```python
from build123d import *

# Parameters (mm, degrees)
F3_R     = 1.55
F4_DEPTH = 21.928203
F7_DEPTH = 4


with BuildPart() as f2:
    # F1 (on Front) → F2 (revolve)
    with BuildSketch(Plane.XZ):
        with BuildLine():
            Line((-4, -6.928203), (-4, -13.928203))
            Line((-4, -13.928203), (0, -13.928203))
            Line((0, -13.928203), (0, 8))
            ThreePointArc((0, 8), (-7.727407, 2.070552), (-4, -6.928203))
        make_face()
    revolve(axis=Axis((0, 0, -6.658787), (0, 0, -1)))

    # F3 (on face) → F4 (cut, through all)
    with BuildSketch(Plane(origin=(0, 0, -13.928203), x_dir=(1, 0, 0), z_dir=(0, 0, -1))):
        Circle(F3_R)
    extrude(amount=-F4_DEPTH, mode=Mode.SUBTRACT)

    # F6 (on offset) → F7 (cut)
    with BuildSketch(Plane.XY.offset(8)):
        Polygon((0.251373, -3.240264), (2.931837, -1.402437), (2.680465, 1.837827), (-0.251373, 3.240264), (-2.931837, 1.402437), (-2.680465, -1.837827), align=None)
    extrude(amount=-F7_DEPTH, mode=Mode.SUBTRACT)

    # F8 (on Front) → F9 (revolve)
    with BuildSketch(Plane.XZ):
        with BuildLine():
            Line((3.934291, -11.928251), (3.948121, -13.928203))
            Line((3.948121, -13.928203), (5.948121, -13.928203))
            ThreePointArc((5.948121, -13.928203), (5.227793, -12.639651), (3.934291, -11.928251))
        make_face()
    revolve(axis=Axis((0, 0, -6.658787), (0, 0, -1)))


solid = f2.part
```
Here's how the part is built. I have some questions about the finished solid (model axes, mm). A direction names the side the tool comes from. Give positions to 0.01 mm unless a question says otherwise; leave off trailing zeros. Use a Markdown table: item, result. Add a question column.
1. If we mould it in two halves opening along X, with no side actions, what happens to faces 1 (the cylindrical face through (0.867, -3.905, -9.471)), 2 (the flat face through (-1.573, 2.334, 5.769)), 3 (the flat face through (-2.808, -0.195, 5.77)), 4 (the flat face through (-1.24, -1.24, -13.928))? For each: +X half, -X half, draft (parallel to the pull), parting line (faces both ways), or undercut.
2. On a 3-axis mill with a long thin cutter (end or side, diameter ignored), from which of +Z, -Z, +X, -X, +Y, -Y can I reach the whole of each face in a straight line? I mean faces 5 (the cylindrical face through (0.715, 1.375, -5.09)), 6 (the flat face through (-1.235, -2.529, 5.769)). Say none if no direction works.
3. For pin 1 Ø1.8 at (x, y) = (-1, 1) entering from +Z; pin 2 Ø4 at (x, y) = (0, 6.5) entering from +Z; pin 3 Ø1.5 at (y, z) = (5, -5) entering from +X, each with a flat end and sliding along its axis, tell me the tip position at first contact or that it passes through.
4. I need wall thicknesses on probe 1 along X at (y, z) = (0, -9); probe 2 along Z at (x, y) = (1.25, 5.25); probe 3 along Y at (x, z) = (-0.75, -9.5). Which ranges of each line are inside material? Lowest first, please. Write a range as from..to.
Results list:
| question | item | result |
|---|---|---|
| 1 | face 1 | parting line |
| 1 | face 2 | undercut |
| 1 | face 3 | undercut |
| 1 | face 4 | draft |
| 2 | face 5 | +Z, -Z |
| 2 | face 6 | +Z |
| 3 | pin 1 | stops at z = 4 |
| 3 | pin 2 | stops at z = 6.61 |
| 3 | pin 3 | stops at x = 4.9 |
| 4 | probe 1 | x = -4..-1.55, 1.55..4 |
| 4 | probe 2 | z = -13.93..-12.82, -5.91..5.91 |
| 4 | probe 3 | y = -3.93..-1.36, 1.36..3.93 |
